Geometry: see drawing. Coordinates: mm, zero at the bounding-box minimum. A direction names the side the tool comes from. Coordinates: 2 decimals unless noted, no trailing zeros. Order: outer loops, then holes, each group sorted by start corner. A loop starts at its lowest first (then second) coordinate and runs counter-clockwise, first axis right, second up.
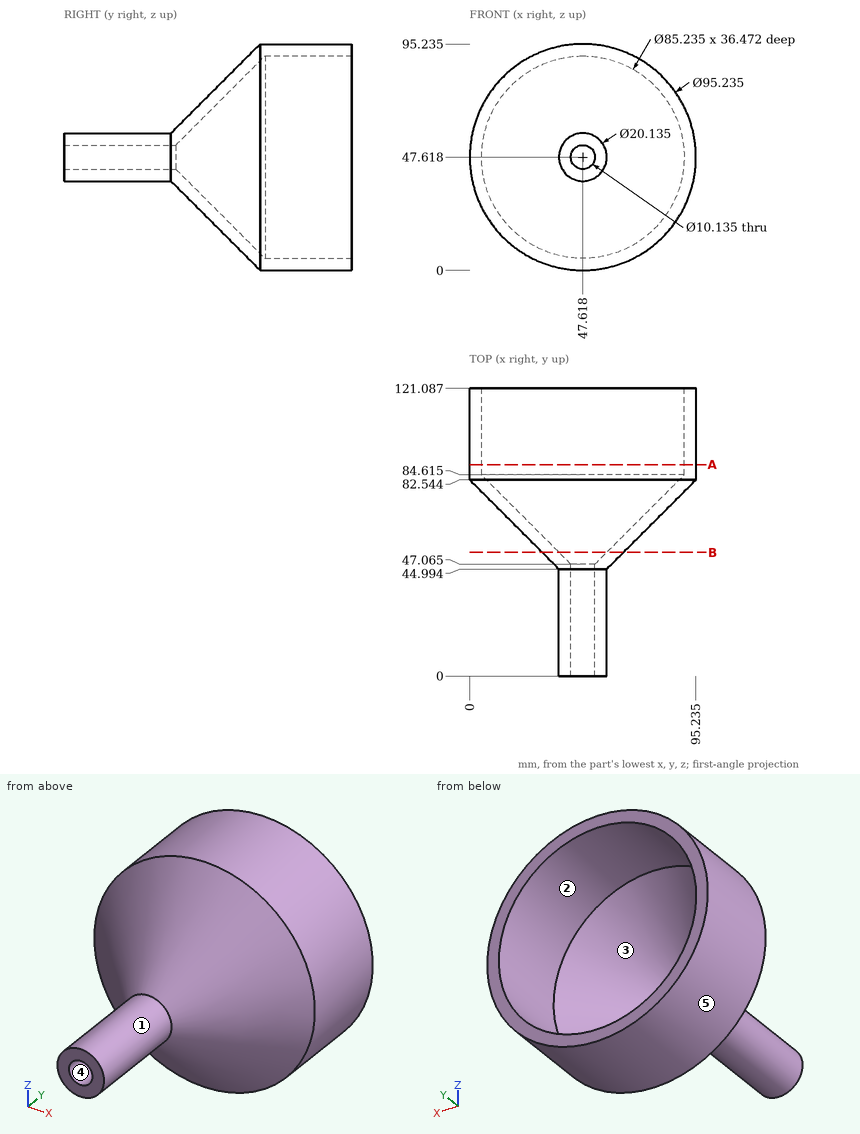
Item 1: Cut plane B-B on y = 52. Return loops of the section in (x, z) (1 decimal).
Response values:
outline: circle Ø34.1 at (47.6, 47.6); hole circle Ø20 at (47.6, 47.6)
Item 2: Pin query (flat end, axial travel): pin 1 Ø6 at (x, z) = (18.5, 46) entering from -Y; pin 2 Ø11.5 at (x, z) = (47.62, 47.62) entering from +Y; pin 3 Ø5 at (x, z) = (74.5, 38.5) entering from -Y. Return the tip coordinate at first contact, or that it passes through.
Response values:
pin 1: stops at y = 61.09
pin 2: stops at y = 47.75
pin 3: stops at y = 60.81
Item 3: Access query for the marked faces 1 and 2. Directions: +Z, -Z, +X, -X, +Y, -Y. A direction counts if a zero-diameter tool reaches every point of the face in a straight line with its end or side. Return the directions, or none.
Response values:
face 1: -Y
face 2: +Y
Item 4: Draft query along X for the marked faces 3, 4 and 5. Return one class per face: pulls with the +X half, pulls with the -X half, needs draft (parallel to the pull), parting line crosses it, or undercut.
Response values:
face 3: undercut
face 4: undercut
face 5: parting line crosses it
Item 5: Cut plane A-A on y = 89. Return loops of the section in (x, z) (1 decimal).
Response values:
outline: circle Ø95.2 at (47.6, 47.6); hole circle Ø85.2 at (47.6, 47.6)
Item 6: Ray query, probe 1 along Z at (x, y) = (47.5, 97) (1 decimal); probe 2 along X at (y, z) = (111, 50.5); probe 3 along X at (y, z) = (88, 82) (1 decimal). Return the intervals inside material, ascending.
Response values:
probe 1: z = 0 to 5, 90.2 to 95.2
probe 2: x = 0.09 to 5.1, 90.14 to 95.15
probe 3: x = 14.7 to 22.4, 72.8 to 80.6
